from build123d import *

# Parameters (mm, degrees)
BOSS_EXTRUDE1_DEPTH = 4.51
CUT_EXTRUDE1_DEPTH  = 4.2
SKETCH5_R           = 1
CUT_EXTRUDE2_DEPTH  = 4.1
SKETCH6_R           = 2
BOSS_EXTRUDE2_DEPTH = 1
SKETCH7_R           = 0.9
CUT_EXTRUDE3_DEPTH  = 1
SKETCH8_R           = 0.5
CUT_EXTRUDE4_DEPTH  = 1
SKETCH9_R           = 0.5
SKETCH9_R_2         = 0.985
SKETCH9_R_3         = 0.675
CUT_EXTRUDE5_DEPTH  = 1
SKETCH10_R          = 0.9
SKETCH10_R_2        = 0.75
BOSS_EXTRUDE3_DEPTH = 0.5
SKETCH11_W          = 3
SKETCH11_H          = 8.25
SKETCH11_W_2        = 2.8
SKETCH11_H_2        = 6.6
CUT_EXTRUDE6_DEPTH  = 0.6
SKETCH12_W          = 6.5
SKETCH12_H          = 2.5
CUT_EXTRUDE7_DEPTH  = 0.6
SKETCH15_W          = 2.5
SKETCH15_H          = 6.6
SKETCH15_W_2        = 2
SKETCH15_H_2        = 4
CUT_EXTRUDE8_DEPTH  = 0.6
SKETCH16_R          = 0.65
BOSS_EXTRUDE4_DEPTH = 4.2
SKETCH17_R          = 0.55
BOSS_EXTRUDE5_DEPTH = 3.5


with BuildPart() as part:
    # Sketch2 → Boss-Extrude1 (new body)
    with BuildSketch(Plane.XY):
        with BuildLine():
            ThreePointArc((-13.711599695, 0.852101617), (-13.847357447, 0.940933533), (-13.9, 1.09439375))
            Line((-13.9, 1.09439375), (-13.9, 24.20560625))
            ThreePointArc((-13.9, 24.20560625), (-13.847357447, 24.359066467), (-13.711599695, 24.447898383))
            Line((-13.711599695, 24.447898383), (-10.481270444, 25.269168531))
            ThreePointArc((-10.481270444, 25.269168531), (-10.359031781, 25.292262196), (-10.234871665, 25.3))
            Line((-10.234871665, 25.3), (-3.665128335, 25.3))
            ThreePointArc((-3.665128335, 25.3), (-3.540968219, 25.292262196), (-3.418729556, 25.269168531))
            Line((-3.418729556, 25.269168531), (-0.188400305, 24.447898383))
            ThreePointArc((-0.188400305, 24.447898383), (-0.052642553, 24.359066467), (0, 24.20560625))
            Line((0, 24.20560625), (0, 1.09439375))
            ThreePointArc((0, 1.09439375), (-0.052642553, 0.940933533), (-0.188400305, 0.852101617))
            Line((-0.188400305, 0.852101617), (-3.418729556, 0.030831469))
            ThreePointArc((-3.418729556, 0.030831469), (-3.540968219, 0.007737804), (-3.665128335, 0))
            Line((-3.665128335, 0), (-10.234871665, 0))
            ThreePointArc((-10.234871665, 0), (-10.359031781, 0.007737804), (-10.481270444, 0.030831469))
            Line((-10.481270444, 0.030831469), (-13.711599695, 0.852101617))
        make_face()
    extrude(amount=BOSS_EXTRUDE1_DEPTH)

    # Sketch4 → Cut-Extrude1 (cut)
    with BuildSketch(Plane(origin=(0, 0, 0), x_dir=(-1, 0, 0), z_dir=(0, 0, -1))):
        with BuildLine():
            Line((13.3, 1.366545), (13.3, 23.933455))
            Line((13.3, 23.933455), (10.333431177, 24.687667412))
            ThreePointArc((10.333431177, 24.687667412), (10.284535712, 24.696904878), (10.234871665, 24.7))
            Line((10.234871665, 24.7), (3.665128335, 24.7))
            ThreePointArc((3.665128335, 24.7), (3.615464288, 24.696904878), (3.566568823, 24.687667412))
            Line((3.566568823, 24.687667412), (0.6, 23.933455))
            Line((0.6, 23.933455), (0.6, 1.366545))
            Line((0.6, 1.366545), (3.566568823, 0.612332588))
            ThreePointArc((3.566568823, 0.612332588), (3.615464288, 0.603095122), (3.665128335, 0.6))
            Line((3.665128335, 0.6), (10.234871665, 0.6))
            ThreePointArc((10.234871665, 0.6), (10.284535712, 0.603095122), (10.333431177, 0.612332588))
            Line((10.333431177, 0.612332588), (13.3, 1.366545))
        make_face()
    extrude(amount=-CUT_EXTRUDE1_DEPTH, mode=Mode.SUBTRACT)

    # Sketch5 → Cut-Extrude2 (cut)
    with BuildSketch(Plane(origin=(0, 0, 4.2), x_dir=(-1, 0, 0), z_dir=(0, 0, -1))):
        with Locations((6.95, 6.6)):
            Circle(SKETCH5_R)
    extrude(amount=-CUT_EXTRUDE2_DEPTH, mode=Mode.SUBTRACT)

    # Sketch6 → Boss-Extrude2 (add)
    with BuildSketch(Plane(origin=(0, 0, 4.2), x_dir=(-1, 0, 0), z_dir=(0, 0, -1))):
        with BuildLine():
            Line((10.333431177, 0.612332588), (7.641436182, 4.197518781))
            ThreePointArc((7.641436182, 4.197518781), (9.050983212, 5.245057365), (9.423767329, 6.961213511))
            Line((9.423767329, 6.961213511), (13.3, 8.366545))
            Line((13.3, 8.366545), (13.3, 8.898391577))
            Line((13.3, 8.898391577), (9.301519142, 7.448738903))
            ThreePointArc((9.301519142, 7.448738903), (6.95, 9.1), (4.598480858, 7.448738903))
            Line((4.598480858, 7.448738903), (0.6, 8.898391577))
            Line((0.6, 8.898391577), (0.6, 8.366545))
            Line((0.6, 8.366545), (4.476232671, 6.961213511))
            ThreePointArc((4.476232671, 6.961213511), (4.849016788, 5.245057365), (6.258563818, 4.197518781))
            Line((6.258563818, 4.197518781), (3.566568823, 0.612332588))
            ThreePointArc((3.566568823, 0.612332588), (3.615464288, 0.603095122), (3.665128335, 0.6))
            Line((3.665128335, 0.6), (4.182568645, 0.6))
            Line((4.182568645, 0.6), (6.813404294, 4.103734467))
            ThreePointArc((6.813404294, 4.103734467), (6.95, 4.1), (7.086595706, 4.103734467))
            Line((7.086595706, 4.103734467), (9.717431355, 0.6))
            Line((9.717431355, 0.6), (10.234871665, 0.6))
            ThreePointArc((10.234871665, 0.6), (10.284535712, 0.603095122), (10.333431177, 0.612332588))
        make_face()
        with Locations((6.95, 6.6)):
            Circle(SKETCH6_R, mode=Mode.SUBTRACT)
    extrude(amount=BOSS_EXTRUDE2_DEPTH)

    # Sketch7 → Cut-Extrude3 (cut)
    with BuildSketch(Plane(origin=(0, 0, 4.2), x_dir=(-1, 0, 0), z_dir=(0, 0, -1))):
        with Locations((6.95, 13.6)):
            Circle(SKETCH7_R)
    extrude(amount=-CUT_EXTRUDE3_DEPTH, mode=Mode.SUBTRACT)

    # Sketch8 → Cut-Extrude4 (cut)
    with BuildSketch(Plane(origin=(0, 0, 4.2), x_dir=(-1, 0, 0), z_dir=(0, 0, -1))):
        with Locations(Location((6.95, 24.2, 0), (0, 0, 90))):
            Circle(SKETCH8_R)
    extrude(amount=-CUT_EXTRUDE4_DEPTH, mode=Mode.SUBTRACT)

    # Sketch9 → Cut-Extrude5 (cut)
    with BuildSketch(Plane(origin=(0, 0, 4.2), x_dir=(-1, 0, 0), z_dir=(0, 0, -1))):
        with Locations((5.95, 19.1)):
            Circle(SKETCH9_R)
        with Locations((9.95, 18.3)):
            Circle(SKETCH9_R_2)
        with Locations((2.6, 17.35)):
            Circle(SKETCH9_R_3)
    extrude(amount=-CUT_EXTRUDE5_DEPTH, mode=Mode.SUBTRACT)

    # Sketch10 → Boss-Extrude3 (add)
    with BuildSketch(Plane(origin=(0, 0, 4.2), x_dir=(-1, 0, 0), z_dir=(0, 0, -1))):
        with Locations((2.6, 17.35)):
            Circle(SKETCH10_R)
        with Locations((2.6, 17.35)):
            Circle(SKETCH10_R_2, mode=Mode.SUBTRACT)
        with BuildLine():
            ThreePointArc((6.348411752, 18.18279333), (6.008413842, 20.098292454), (5.447334993, 18.235518716))
            ThreePointArc((5.447334993, 18.235518716), (5.618228279, 18.28074575), (5.573001245, 18.451639037))
            ThreePointArc((5.573001245, 18.451639037), (5.993810381, 19.84871934), (6.248808814, 18.412094997))
            ThreePointArc((6.248808814, 18.412094997), (6.183959449, 18.247642694), (6.348411752, 18.18279333))
        make_face()
        with BuildLine():
            ThreePointArc((10.652922784, 17.227125511), (10.778596901, 19.279074709), (8.775669457, 18.815856457))
            ThreePointArc((8.775669457, 18.815856457), (8.827006943, 18.684082171), (8.95878123, 18.735419658))
            ThreePointArc((8.95878123, 18.735419658), (10.649394907, 19.126408914), (10.543316985, 17.394417378))
            ThreePointArc((10.543316985, 17.394417378), (10.514473951, 17.255968545), (10.652922784, 17.227125511))
        make_face()
    extrude(amount=BOSS_EXTRUDE3_DEPTH)

    # Sketch11 → Cut-Extrude6 (cut)
    with BuildSketch(Plane(origin=(0, 0, 0), x_dir=(0, 0, -1), z_dir=(1, 0, 0))):
        with Locations((-1.5, 18.175)):
            Rectangle(SKETCH11_W, SKETCH11_H)
        with Locations((-1.4, 7.3)):
            Rectangle(SKETCH11_W_2, SKETCH11_H_2)
    extrude(amount=-CUT_EXTRUDE6_DEPTH, mode=Mode.SUBTRACT)

    # Sketch12 → Cut-Extrude7 (cut)
    with BuildSketch(Plane.XZ):
        with Locations((-6.95, 1.25)):
            Rectangle(SKETCH12_W, SKETCH12_H)
    extrude(amount=-CUT_EXTRUDE7_DEPTH, mode=Mode.SUBTRACT)

    # Sketch15 → Cut-Extrude8 (cut)
    with BuildSketch(Plane.ZY.offset(13.9)):
        with Locations((1.25, 7.3)):
            Rectangle(SKETCH15_W, SKETCH15_H)
        with Locations((1, 20)):
            Rectangle(SKETCH15_W_2, SKETCH15_H_2)
    extrude(amount=-CUT_EXTRUDE8_DEPTH, mode=Mode.SUBTRACT)

    # Sketch16 → Boss-Extrude4 (add)
    with BuildSketch(Plane(origin=(0, 0, 4.2), x_dir=(-1, 0, 0), z_dir=(0, 0, -1))):
        with Locations((1.112347538, 23.533455)):
            Circle(SKETCH16_R)
        with Locations((1.112347538, 12.75)):
            Circle(SKETCH16_R)
        with Locations((1.112347538, 1.766545)):
            Circle(SKETCH16_R)
        with Locations((12.787652462, 1.766545)):
            Circle(SKETCH16_R)
        with Locations((12.787652462, 12.75)):
            Circle(SKETCH16_R)
        with Locations((12.787652462, 23.533455)):
            Circle(SKETCH16_R)
    extrude(amount=BOSS_EXTRUDE4_DEPTH)

    # Sketch17 → Boss-Extrude5 (add)
    with BuildSketch(Plane(origin=(0, 0, 0), x_dir=(-1, 0, 0), z_dir=(0, 0, -1))):
        with Locations(Location((1.112347538, 12.75, 0), (0, 0, 180))):
            Circle(SKETCH17_R)
        with Locations(Location((1.112347538, 23.533455, 0), (0, 0, 180))):
            Circle(SKETCH17_R)
        with Locations(Location((1.112347538, 1.766545, 0), (0, 0, 180))):
            Circle(SKETCH17_R)
        with Locations(Location((12.787652462, 1.766545, 0), (0, 0, 180))):
            Circle(SKETCH17_R)
        with Locations(Location((12.787652462, 12.75, 0), (0, 0, 180))):
            Circle(SKETCH17_R)
        with Locations(Location((12.787652462, 23.533455, 0), (0, 0, 180))):
            Circle(SKETCH17_R)
    extrude(amount=BOSS_EXTRUDE5_DEPTH)


solid = part.part
Geometry: final body of the model. Coordinates: model frame, mm. A direction names the side the tool comes from. Round coordinates to 2 decimals unless told otherwise and drop trailing zeros. Order: outer loops, then holes, each group sorted by start corner. A loop starts at its lowest first (then second) coordinate and runs counter-clockwise, first axis right, second up. Notation, with made-up numbers: (-22, 5) -> (-5, 5) arc R15 ccw to (-5, 16) -> close; hole circle Ø4 at (66.25, -16.5). An arc over 180 degrees is marked (long way). Put each result on its own line as item: value. Start each with the question number.
Q1. Reachability of faces 5 (the cylindrical face through (-6.928, 23.7, 4.353)), 6 (the cylindrical face through (-5.97, 19.85, 3.95)) from +Z, -Z, +X, -X, +Y, -Y: full face, straight path, thin tool, end or side. Return the list, or none.
Q2. Section A-A on y = 6.6. Return the cut outline in (x, z), and give its area (3 significant figures).
Q3. Pull-direction query (X, two-part tool) for faces 1 (the flat face through (-13, 2, -3.5)), 2 (the cylindrical face through (-12.284, 2.177, 2.129)), 3 (the flat face through (-1.781, 0.447, 2.223)), 4 (the cylindrical face through (-0.859, 2.254, -1.726)); classes: +X half, -X half, draft (parallel to the pull), parting line (faces both ways), or undercut.
Q4. Section C-C on z = 0.25. Give the number of separate pieces and of enclosed holes in the cut face, and give its area (3 significant figures).
Q5. Section D-D on y = 21. Return the cut outline in (x, z).
Q6. First-contact query: pin 1 (0.7 mm diameter, centred on x = -0.5, z = 2, fed in from -Y); pin 2 (1.1 mm diameter, centred on x = -8, y = 2.5, fed in from -Z); pin 3 (1.1 mm diameter, centred on x = -2.6, y = 17.35, fed in from -Z); pin 4 (1.5 mm diameter, centred on x = -12.5, y = 17.5, fed in from -Z). Flat tips, straight axial feed; report the tip coordinate or a pass-through.
Q7. Line query: probe 1 along X at (y, z) = (6.75, 4); probe 2 along X at (y, z) = (19.1, 4.1); probe 3 along Y at (x, z) = (-1, -2.75). Output: solid intervals per line, ascending.
Q8. Section B-B on x = -2.6. Return the cut outline in (y, z) (3 decimals).
Ans:
1. face 5: +Z, -Z
1. face 6: -Z
2. outline: (-13.9, 2.5) -> (-13.3, 2.5) -> (-13.3, 4.2) -> (-9.45, 4.2) -> (-9.45, 3.2) -> (-8.95, 3.2) -> (-8.95, 4.2) -> (-7.95, 4.2) -> (-7.95, 4.51) -> (-13.9, 4.51) -> close; (-5.95, 4.2) -> (-4.95, 4.2) -> (-4.95, 3.2) -> (-4.45, 3.2) -> (-4.45, 4.2) -> (-0.6, 4.2) -> (-0.6, 2.8) -> (0, 2.8) -> (0, 4.51) -> (-5.95, 4.51) -> close
2. area: 6.55 mm2
3. face 1: draft
3. face 2: undercut
3. face 3: +X half
3. face 4: undercut
4. separate pieces: 5
4. enclosed holes: 0
4. area: 31.9 mm2
5. outline: (-13.9, 2) -> (-13.3, 2) -> (-13.3, 4.2) -> (-0.6, 4.2) -> (-0.6, 3) -> (0, 3) -> (0, 4.51) -> (-13.9, 4.51) -> close
6. pin 1: stops at y = 0.68
6. pin 2: stops at z = 3.2
6. pin 3: passes through
6. pin 4: stops at z = 4.2
7. probe 1: x = -13.9 to -13.3, -9.45 to -8.94, -4.96 to -4.45, -0.6 to 0
7. probe 2: x = -13.9 to -13.3, -10.95 to -10.68, -9.22 to -8.95, -6.95 to -6.7, -5.2 to -4.95, -0.6 to 0
7. probe 3: y = 1.23 to 2.3, 12.21 to 13.29, 23 to 24.07
8. outline: (0.239, 0) -> (0.858, 0) -> (0.858, 4.2) -> (7.641, 4.2) -> (7.641, 3.2) -> (8.173, 3.2) -> (8.173, 4.2) -> (16.45, 4.2) -> (16.45, 3.7) -> (16.6, 3.7) -> (16.6, 4.2) -> (16.675, 4.2) -> (16.675, 4.51) -> (0.239, 4.51) -> close; (18.025, 4.2) -> (18.1, 4.2) -> (18.1, 3.7) -> (18.25, 3.7) -> (18.25, 4.2) -> (24.442, 4.2) -> (24.442, 0) -> (25.061, 0) -> (25.061, 4.51) -> (18.025, 4.51) -> close
